Here's the drawing with two shaded views (mm, measured from the low corner). I have some questions. Coordinates: 2 decimals unless noted, no trailing zeros. Write each loop counter-clockwise with the first axis right and the second up, starting at its lowest first coordinate (ties: lowest second). Pieces come first, ordered by that corner, then holes.
Item 1: If we section it at B-B (z = 11.45): Please give me the cut outline in (x, y), then the cut area to 3 significant figures.
Item 2: If I drill on line 1 (Z direction, x = 5, y = 1.6); line 2 (X direction, y = 4.75, z = 22); line 3 (Z direction, x = 5.75, y = 3.75), over which ranges is the centre line in solid material (lowest first)?
Item 3: If we section it at A-A (x = 5): Please give me the cut outline in (y, z).
Item 4: We'd pull the mould along X, two halves only. Please class the marked faces 1, 2, 3 and 4: +X half, -X half, draft (parallel to the pull), parting line (faces both ways), or undercut.
Item 5: If we section it at C-C (y = 2.5): Please give me the cut outline in (x, z), then the cut area to 3 significant figures.
Item 6: If we section it at D-D (z = 16.8): Please give me the cut outline in (x, y).
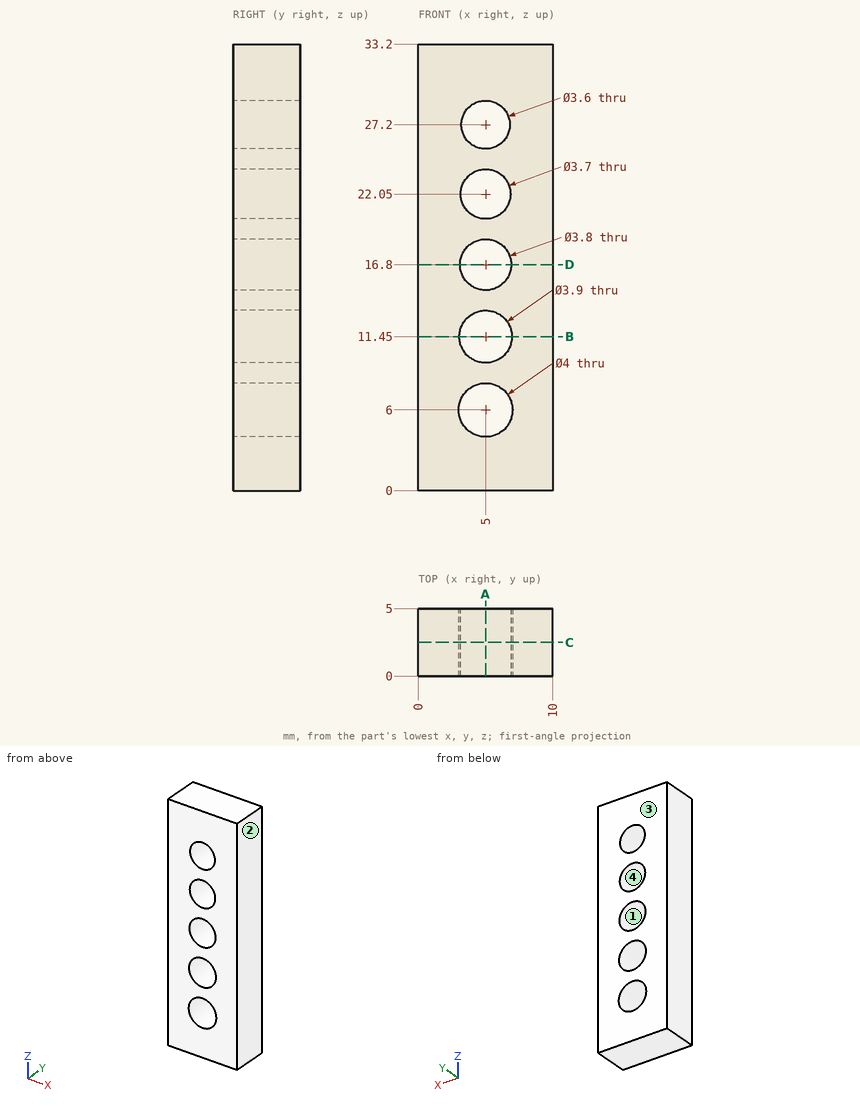
Answer list:
1. outline: (0, 0) - (3.05, 0) - (3.05, 5) - (0, 5) - close; (6.95, 0) - (10, 0) - (10, 5) - (6.95, 5) - close
1. area: 30.5 mm2
2. line 1: z = 0 to 4, 8 to 9.5, 13.4 to 14.9, 18.7 to 20.2, 23.9 to 25.4, 29 to 33.2
2. line 2: x = 0 to 3.15, 6.85 to 10
2. line 3: z = 0 to 4.15, 7.85 to 9.65, 13.25 to 15.05, 18.55 to 20.36, 23.74 to 25.56, 28.84 to 33.2
3. outline: (0, 0) - (5, 0) - (5, 4) - (0, 4) - close; (0, 8) - (5, 8) - (5, 9.5) - (0, 9.5) - close; (0, 13.4) - (5, 13.4) - (5, 14.9) - (0, 14.9) - close; (0, 18.7) - (5, 18.7) - (5, 20.2) - (0, 20.2) - close; (0, 23.9) - (5, 23.9) - (5, 25.4) - (0, 25.4) - close; (0, 29) - (5, 29) - (5, 33.2) - (0, 33.2) - close
4. face 1: undercut
4. face 2: +X half
4. face 3: draft
4. face 4: undercut
5. outline: (0, 0) - (10, 0) - (10, 33.2) - (0, 33.2) - close; hole circle Ø4 at (5, 6); hole circle Ø3.9 at (5, 11.45); hole circle Ø3.8 at (5, 16.8); hole circle Ø3.7 at (5, 22.05); hole circle Ø3.6 at (5, 27.2)
5. area: 275 mm2
6. outline: (0, 0) - (3.1, 0) - (3.1, 5) - (0, 5) - close; (6.9, 0) - (10, 0) - (10, 5) - (6.9, 5) - close
